```python
from build123d import *

# Parameters (mm, degrees)
F1_DEPTH = 76.2
F2_W     = 31.75
F2_H     = 31.75
F3_DEPTH = 19.05
F4_R     = 15.875
F5_DEPTH = 25.4
F6_W     = 171.45
F6_H     = 50.8
F6_R     = 15.875
F7_DEPTH = 25.4


with BuildPart() as f1:
    # F0 (on Front) → F1 (new body, symmetric)
    with BuildSketch(Plane.XZ):
        Polygon((38.1, 53.975), (-38.1, 53.975), (-38.1, 73.025), (-69.85, 73.025), (-69.85, 53.975), (-69.85, 31.75), (69.85, 31.75), (69.85, 53.975), (69.85, 73.025), (38.1, 73.025), align=None)
    extrude(amount=F1_DEPTH, both=True)

    # F2 (on face) → F3 (join)
    with BuildSketch(Plane.XY.offset(73.025)):
        with Locations((53.975, 60.325)):
            Rectangle(F2_W, F2_H)
        with Locations((53.975, -60.325)):
            Rectangle(F2_W, F2_H)
        with Locations((-53.975, 60.325)):
            Rectangle(F2_W, F2_H)
        with Locations((-53.975, -60.325)):
            Rectangle(F2_W, F2_H)
    extrude(amount=F3_DEPTH)

    # F4 (on face) → F5 (cut)
    with BuildSketch(Plane.XY.offset(53.975)):
        Circle(F4_R)
    extrude(amount=-F5_DEPTH, mode=Mode.SUBTRACT)

    # F6 (on face) → F7 (join)
    with BuildSketch(Plane(origin=(0, 0, 31.75), x_dir=(1, 0, 0), z_dir=(0, 0, -1))):
        Polygon((127, 76.2), (-127, 76.2), (-127, 25.4), (-85.725, 25.4), (85.725, 25.4), (127, 25.4), align=None)
        Rectangle(F6_W, F6_H)
        Circle(F6_R, mode=Mode.SUBTRACT)
        Polygon((85.725, -25.4), (-85.725, -25.4), (-127, -25.4), (-127, -76.2), (127, -76.2), (127, -25.4), align=None)
    extrude(amount=F7_DEPTH)


solid = f1.part
```
Read the model definition and answer for the solid it produces. Units are mm, in the model's axes. A direction names the side the tool comes from. Round coordinates to 2 decimals unless told otherwise and drop trailing zeros. Write each loop counter-clockwise with the first axis right and the second up, starting at its lowest first coordinate (ties: lowest second). Pieces come first, ordered by that corner, then holes. Notation, with made-up numbers: (36.5, -31.75) -> (94.5, -31.75) arc R19 cw to (94.5, -22.75) -> close; hole circle Ø10 at (-9, -39). An arc over 180 degrees is marked (long way). Answer in a Markdown table with one row per item. Add a question column.
1) Find section C-C, the plane x = 0. Determine the outline of the cut face in (y, z) (3 decimals), and give its area (3 significant figures).
2) Given P1, Ø23, axis at x = -16.5, y = 20, coming from the +Z side (3 decimals); P2, Ø6, axis at y = -18, z = 65.5, coming from the +X side; P3, Ø19, axis at y = -14, z = 68, coming from the -X side; P4, Ø12, axis at x = 35, z = 63.5, coming from the -Y side, each flat-ended and moving along its own axis, determine where each tip first touches the part or whether it passes through.
3) Which of the six approach directions +Z, -Z, +X, -X, +Y, -Y give full straight-line access (tool end or side, diameter ignored) to faces 4 (the face through (-38.1, -1, 69)), 5 (the face through (-80, -1, 31.75)), 6 (the face through (54, 44.45, 82)), 7 (the face through (-107, -25.4, 19))?
4) Determine the mould class of faces 1 (the face through (-54, -1, 73.025)), 2 (the face through (-54, -60, 92.075)), 3 (the face through (-2, 76.2, 40)) for opening direction Y: pulls with the +Y half, pulls with the -Y half, needs draft (parallel to the pull), parting line crosses it, or undercut.
5) Find section B-B, the plane y = 0. Determine the outline of the cut face in (x, z) (3 decimals), and give its area (3 significant figures).
6) Consider line 1 (Y direction, x = 0, z = 38) (3 decimals); line 2 (Y direction, x = 115.5, z = 29.5); line 3 (X direction, y = -0.5, z = 48). Determine where each line is inside the solid, lowest interval first.
7) Find section D-D, the plane y = 21.5. Determine the outline of the cut face in (x, z) (3 decimals), and give its area (3 significant figures).
8) Find section A-A, the plane z = 78. Determine the outline of the cut face in (x, y), and give its area (3 significant figures).
Findings below:
| question | item | result |
|---|---|---|
| 1 | outline | (-76.2, 6.35) -> (-15.875, 6.35) -> (-15.875, 53.975) -> (-76.2, 53.975) -> close; (15.875, 6.35) -> (76.2, 6.35) -> (76.2, 53.975) -> (15.875, 53.975) -> close |
| 1 | area | 5,750 mm² |
| 2 | P1 | z = 53.975 |
| 2 | P2 | x = 69.85 |
| 2 | P3 | x = -69.85 |
| 2 | P4 | y = -76.2 |
| 3 | face 4 | +Z, +Y, -Y |
| 3 | face 5 | +Z, -X, +Y, -Y |
| 3 | face 6 | +Z, +X, -X |
| 3 | face 7 | +Z, -Z, -X |
| 4 | face 1 | undercut |
| 4 | face 2 | needs draft |
| 4 | face 3 | pulls with the +Y half |
| 5 | outline | (-85.725, 6.35) -> (-15.875, 6.35) -> (-15.875, 53.975) -> (-38.1, 53.975) -> (-38.1, 73.025) -> (-69.85, 73.025) -> (-69.85, 31.75) -> (-85.725, 31.75) -> close; (15.875, 6.35) -> (85.725, 6.35) -> (85.725, 31.75) -> (69.85, 31.75) -> (69.85, 73.025) -> (38.1, 73.025) -> (38.1, 53.975) -> (15.875, 53.975) -> close |
| 5 | area | 7,160 mm² |
| 6 | line 1 | -76.2 to -15.875, 15.875 to 76.2 |
| 6 | line 2 | -76.2 to -25.4, 25.4 to 76.2 |
| 6 | line 3 | -69.85 to -15.87, 15.87 to 69.85 |
| 7 | outline | (-85.725, 6.35) -> (85.725, 6.35) -> (85.725, 31.75) -> (69.85, 31.75) -> (69.85, 73.025) -> (38.1, 73.025) -> (38.1, 53.975) -> (-38.1, 53.975) -> (-38.1, 73.025) -> (-69.85, 73.025) -> (-69.85, 31.75) -> (-85.725, 31.75) -> close |
| 7 | area | 8,670 mm² |
| 8 | outline | (-69.85, -76.2) -> (-38.1, -76.2) -> (-38.1, -44.45) -> (-69.85, -44.45) -> close; (-69.85, 44.45) -> (-38.1, 44.45) -> (-38.1, 76.2) -> (-69.85, 76.2) -> close; (38.1, -76.2) -> (69.85, -76.2) -> (69.85, -44.45) -> (38.1, -44.45) -> close; (38.1, 44.45) -> (69.85, 44.45) -> (69.85, 76.2) -> (38.1, 76.2) -> close |
| 8 | area | 4,030 mm² |
